```python
from build123d import *

# Parameters (mm, degrees)
SKETCH1_W                 = 7
SKETCH1_H                 = 5
BOSS_EXTRUDE1_DEPTH       = 4
M3X0_5_TAPPED_HOLE1_D     = 2.5
M3X0_5_TAPPED_HOLE1_DEPTH = 8.5
M3X0_5_TAPPED_HOLE1_TIP   = 0.751075774
SKETCH6_W                 = 4
SKETCH6_H                 = 5
CUT_EXTRUDE1_DEPTH        = 2
CHAMFER1_SIZE             = 1


with BuildPart() as part:
    # Sketch1 → Boss-Extrude1 (new body)
    with BuildSketch(Plane.XY):
        with Locations((3.5, 2.5)):
            Rectangle(SKETCH1_W, SKETCH1_H)
    extrude(amount=BOSS_EXTRUDE1_DEPTH)

    # M3x0.5 Tapped Hole1
    with Locations(Plane(origin=(0, 0, 0), x_dir=(-1, 0, 0), z_dir=(0, 0, -1))):
        with Locations((-3.1, 2)):
            Hole(M3X0_5_TAPPED_HOLE1_D / 2, depth=M3X0_5_TAPPED_HOLE1_DEPTH)
            with Locations((0, 0, -(M3X0_5_TAPPED_HOLE1_DEPTH + M3X0_5_TAPPED_HOLE1_TIP / 2))):  # 118° drill point
                Cone(0, M3X0_5_TAPPED_HOLE1_D / 2, M3X0_5_TAPPED_HOLE1_TIP, mode=Mode.SUBTRACT)

    # Sketch6 → Cut-Extrude1 (cut)
    with BuildSketch(Plane.XY.offset(4)):
        with Locations((5, 2.5)):
            Rectangle(SKETCH6_W, SKETCH6_H)
    extrude(amount=-CUT_EXTRUDE1_DEPTH, mode=Mode.SUBTRACT)

    # Chamfer1
    # the kernel refuses this chamfer: 1 mm, written as the material it takes off along each edge
    with BuildSketch(Plane(origin=(-2.571682988, 0, 0), x_dir=(0, -0.027495876610586372, 0.9996219169112968), z_dir=(1, 0, 0))) as chamfer1_piece_1:
        Polygon((CHAMFER1_SIZE * 0.999621916911, -CHAMFER1_SIZE * 0.0274958766106), (-CHAMFER1_SIZE * 0.0274958766106, -CHAMFER1_SIZE * 0.999621916911), (0, 0), align=None)
    extrude(amount=12.143365976, mode=Mode.SUBTRACT)


solid = part.part
```
Could you check a few things on this model? Use its own coordinates, in mm. A direction names the side the tool comes from. Round coordinates to 2 decimals unless told otherwise and drop trailing zeros. Loops run counter-clockwise (first coordinate to the right, second up) from the corner with the lowest first, then second, coordinate; pieces in that order, holes last. Notation, with made-up numbers: M 75.25,14 L 91.25,14 A23 ccw 91.25,24 Z; hole C 32,82.5 d7. An arc over 180 degrees is marked long. Answer as CSV lines item,"result".
1) For pin 1 Ø1.4 at (y, z) = (4, 3.5) entering from +X; pin 2 Ø2 at (x, y) = (5, 2.5) entering from +Z, each with a flat end and sliding along its axis, tell me the tip position at first contact or that it passes through.
From the geometry:
pin 1,"x = 3"
pin 2,"z = 2"
2) Imagine slicing it at C-C on z = 1.8. List the corners of the cut face in (x, y) for me, and give its area (3 significant figures).
From the geometry:
outline,"M 0,0 L 7,0 L 7,5 L 0,5 Z; hole C 3.1,2 d2.5"
area,"30.1 mm^2"
3) Imagine slicing it at B-B on x = 3.1. List the corners of the cut face in (y, z) for me, and give its area (3 significant figures).
From the geometry:
outline,"M 0,1 L 0.75,0.25 L 0.75,2 L 0,2 Z; M 3.25,0 L 5,0 L 5,2 L 3.25,2 Z"
area,"4.53 mm^2"
4) Imagine slicing it at A-A on y = 2. List the corners of the cut face in (x, z) for me.
From the geometry:
outline,"M 0,0 L 1.85,0 L 1.85,4 L 0,4 Z; M 4.35,0 L 7,0 L 7,2 L 4.35,2 Z"
5) Which directions (+Z, -Z, +X, -X, +Y, -Y) give clear straight access to the entire face, cutting with the end or side of a thin tool? Please do faces 5 (the flat face through (3, 4, 3)), 6 (the flat face through (3.5, 3.5, 0)).
From the geometry:
face 5,"+Z, +X, +Y, -Y"
face 6,"-Z, +X, -X, +Y, -Y"
6) If I drill on probe 1 along X at (y, z) = (2, 1.6); probe 2 along Y at (x, z) = (3.1, 1.8); probe 3 along X at (y, z) = (2, 2.15), over which ranges is the centre line in solid material (lowest first)?
From the geometry:
probe 1,"0 to 1.85, 4.35 to 7"
probe 2,"0 to 0.75, 3.25 to 5"
probe 3,"0 to 1.85"
7) We'd pull the mould along Y, two halves only. Please class faces 1 (the flat face through (0, 2, 2)), 2 (the cylindrical face through (1.85, 2.05, 1.58)), 3 (the flat face through (2.7, 5, 1.5)), 4 (the flat face through (3.5, 0.5, 0.5)): released by +Y, released by -Y, zero draft, split by the parting line, or undercut.
From the geometry:
face 1,"zero draft"
face 2,"undercut"
face 3,"released by +Y"
face 4,"released by -Y"
